Work out the finished part from the listing and answer in its coordinate system (mm). A direction names the side the tool comes from. Round coordinates to 2 decimals unless told otherwise and drop trailing zeros. Order: outer loops, then holes, each group sorted by start corner. A loop starts at its lowest first (then second) coordinate and runs counter-clockwise, first axis right, second up. Notation, with made-up numbers: M 80.25,-8.75 L 111.25,-8.75 A17 cw 111.25,3.25 Z; hole C 53,37.25 d1. An arc over 180 degrees is marked long. Return JSON: item names as keys, results as strings.
from build123d import *

# Parameters (mm, degrees)
CHAMFER1_SIZE = 1.25


with BuildPart() as part:
    # Sketch1 → Revolve1 (revolve)
    with BuildSketch(Plane(origin=(0, 0, 0), x_dir=(0, 0, -1), z_dir=(1, 0, 0))):
        with BuildLine():
            Line((0, 0), (0, 85.55))
            Line((0, 85.55), (3.18, 85.55))
            Line((3.18, 85.55), (3.18, 18.522021385))
            ThreePointArc((3.18, 18.522021385), (9.786228155, 7.066556842), (22.86, 5.08))
            Line((22.86, 5.08), (26.67, 1.27))
            Line((26.67, 1.27), (26.67, 0))
            Line((26.67, 0), (0, 0))
        make_face()
    revolve(axis=Axis((0, 0, 0), (0, 1, 0)))

    # Chamfer1
    chamfer1_edges = [part.edges().sort_by_distance(p)[0] for p in [
        (0, 85.55, 3.18),
    ]]
    chamfer(chamfer1_edges, length=CHAMFER1_SIZE)


solid = part.part
Item 1: Find section C-C (y = 66). Determine the outline of the cut face in (x, z).
Output:
{"outline": "C 0,0 d6.36"}
Item 2: Find section B-B (z = 0). Determine the outline of the cut face in (x, y), plus the area to 3 significant figures.
Output:
{"outline": "M -26.67,0 L 26.67,0 L 26.67,1.27 L 22.86,5.08 A15.25 cw 3.18,18.52 L 3.18,84.3 L 1.93,85.55 L -1.93,85.55 L -3.18,84.3 L -3.18,18.52 A15.25 cw -22.86,5.08 L -26.67,1.27 Z", "area": "841 mm^2"}
Item 3: Which of the six approach directions +Z, -Z, +X, -X, +Y, -Y give full straight-line access (tool end or side, diameter ignored) to faces 1 (the flat face through (0, 85.55, 0)), 2 (the cylindrical face through (3.1, 51, 0.7))?
Output:
{"face 1": "+Z, -Z, +X, -X, +Y", "face 2": "+Y"}
Item 4: Find section A-A (x = 0). Determine the outline of the cut face in (y, z).
Output:
{"outline": "M 0,-26.67 L 1.27,-26.67 L 5.08,-22.86 A15.25 cw 18.52,-3.18 L 84.3,-3.18 L 85.55,-1.93 L 85.55,1.93 L 84.3,3.18 L 18.52,3.18 A15.25 cw 5.08,22.86 L 1.27,26.67 L 0,26.67 Z"}
Item 5: Each of these flat-tipped pins is pushed along its axis until it touches: pin 1 (10 mm diameter, centred on x = -6.5, y = 65.5, fed in from -Z); pin 2 (10 mm diameter, centred on x = 12.5, y = 36.5, fed in from -Z); pin 3 (5 mm diameter, centred on y = 24.5, z = -2.5, fed in from +X); pin 4 (1 mm diameter, centred on x = -20, z = -11.5, fed in from +Y). Where does it stop, or does it pass through?
Output:
{"pin 1": "stops at z = -2.8", "pin 2": "passes through", "pin 3": "stops at x = 3.18", "pin 4": "stops at y = 5.08"}
Item 6: Find section D-D (y = 7). Determine the outline of the cut face in (x, z), plus the area to 3 significant figures.
Output:
{"outline": "C 0,0 d19.77", "area": "307 mm^2"}
Item 7: Consider line 1 along Y through (x, z) = (-5.5, 15); line 2 along Y through (x, z) = (0, 13); line 3 along X through (y, z) = (8, -7). Determine where each line is inside the solid, lowest interval first. Write a range as [from, to].
Output:
{"line 1": "y = [0, 4.6]", "line 2": "y = [0, 5.39]", "line 3": "x = [-4.92, 4.92]"}
